Geometry: final body of the model. Coordinates: model frame, mm. A direction names the side the tool comes from. Round coordinates to 2 decimals unless told otherwise and drop trailing zeros. Order: outer loops, then holes, each group sorted by start corner. A loop starts at its lowest first (then second) coordinate and runs counter-clockwise, first axis right, second up. Notation, with made-up numbers: M 88.5,51 L 103.5,51 A12 ccw 103.5,61 Z; hole C 0.5,14.5 d8. An arc over 180 degrees is marked long. Put each result on its own line as item: value. Start each with the question number.
1) Section A-A, the plane y = 3.25. Return loops of the section in (x, z), then the cut area to 3 significant figures.
2) Access query for faces 1 (the flat face through (-10, 3, -16.75)), 2 (the flat face through (-2, 3, -10)), 3 (the flat face through (-10, 3, -2)). Directions: +Z, -Z, +X, -X, +Y, -Y. A direction counts if a zero-diameter tool reaches every point of the face in a straight line with its end or side. Return the directions, or none.
3) Material intervals for probe 1 along X at (y, z) = (2.5, -13.5); probe 2 along Z at (x, y) = (-10, 6.5), sorted ascending. Write a range as [from, to].
4) First-contact query: P1, Ø3, axis at y = 7.5, z = -12.5, coming from the -X side; P2, Ø2, axis at x = -7.5, y = 6, coming from the -Z side; P3, Ø1.5, axis at x = -8, y = 7, coming from the +Z side. Flat tips, straight axial feed; report the tip coordinate or a pass-through.
5) Section D-D, the plane y = 6.5. Return loops of the section in (x, z).
6) Section C-C, the plane z = -13.75. Return loops of the section in (x, y).
7) Draft query along X for faces 4 (the flat face through (-6, 7, -10)), 5 (the flat face through (-18, 3, -10)), 6 (the flat face through (-10, 2, -19)). Return one class per face: pulls with the +X half, pulls with the -X half, needs draft (parallel to the pull), parting line crosses it, or undercut.
8) Section B-B, the plane x = -5.75. Return loops of the section in (y, z), then the cut area to 3 significant figures.
Autodesk Inventor part; units mm, degrees
ref_plane "YZ Plane" through (0, 0, 0) normal (1, 0, 0) x (0, 1, 0)
ref_plane "XZ Plane" through (0, 0, 0) normal (0, 1, 0) x (-1, 0, 0)
ref_plane "XY Plane" through (0, 0, 0) normal (0, 0, 1) x (1, 0, 0)
sketch "Sketch1" plane through (0, 0, 0) normal (0, 1, 0) x (-1, 0, 0)
  line L0 (0, 0) -> (20, 0)
  line L1 (20, 0) -> (20, -20)
  line L2 (20, -20) -> (0, -20)
  line L3 (0, -20) -> (0, 0)
  dimension "d0" = 20
  dimension "d1" = 20
extrude "Extrusion1" add sketch "Sketch1" along normal blind 2
sketch "Sketch2" plane through (0, 2, 0) normal (0, 1, 0) x (1, 0, 0)
  line L0 (0, 20) -> (-20, 20)
  line L1 (-20, 20) -> (-20, 0)
  line L2 (-20, 0) -> (0, 0)
  line L3 (0, 0) -> (0, 20)
  line L4 (-18, 2) -> (-18, 18)
  line L5 (-18, 18) -> (-2, 18)
  line L6 (-2, 18) -> (-2, 2)
  line L7 (-2, 2) -> (-18, 2)
  line L8 (-16.75, 16.75) -> (-16.75, 3.25)
  line L9 (-16.75, 3.25) -> (-3.25, 3.25)
  line L10 (-3.25, 3.25) -> (-3.25, 16.75)
  line L11 (-3.25, 16.75) -> (-16.75, 16.75)
  dimension "d4" = 2
  dimension "d5" = 1.25
extrude "Extrusion2" add sketch "Sketch2" along normal blind 2 contours L4 L5 L6 L7
extrude "Extrusion3" cut sketch "Sketch2" against normal blind 10 contours L11 L10 L9 L8
sketch "Sketch3" plane through (0, 0, 0) normal (0, -1, 0) x (1, 0, 0)
  line L0 (-3.25, -3.25) -> (-3.25, -16.75)
  line L1 (-3.25, -16.75) -> (-16.75, -16.75)
  line L2 (-16.75, -16.75) -> (-16.75, -3.25)
  line L3 (-16.75, -3.25) -> (-3.25, -3.25)
  line L4 (0, -20) -> (-20, -20)
  line L5 (0, 0) -> (0, -20)
  line L6 (-20, 0) -> (0, 0)
  line L7 (-20, -20) -> (-20, 0)
  line L8 (-6, -6) -> (-6, -14)
  line L9 (-6, -14) -> (-14, -14)
  line L10 (-14, -14) -> (-14, -6)
  line L11 (-14, -6) -> (-6, -6)
extrude "Extrusion4" add sketch "Sketch3" against normal up to surface (2 mm away) contours L0 L1 L2 L3
extrude "Extrusion5" add sketch "Sketch3" against normal blind 12.5 contours L8 L9 L10 L11
properties part number "latticeChamberCapv4"
Result sheet:
1. outline: M -18,-18 L -2,-18 L -2,-2 L -18,-2 Z; M -14,-14 L -6,-14 L -6,-6 L -14,-6 Z; hole M -16.75,-16.75 L -3.25,-16.75 L -3.25,-3.25 L -16.75,-3.25 Z
1. area: 138 mm2
2. face 1: +Y
2. face 2: +Z, -Z, +X, +Y
2. face 3: +Z, +X, -X, +Y
3. probe 1: x = [-18, -16.75], [-14, -6], [-3.25, -2]
3. probe 2: z = [-14, -6]
4. P1: stops at x = -14
4. P2: stops at z = -14
4. P3: stops at z = -6
5. outline: M -14,-14 L -6,-14 L -6,-6 L -14,-6 Z
6. outline: M -20,0 L 0,0 L 0,2 L -2,2 L -2,4 L -3.25,4 L -3.25,2 L -6,2 L -6,12.5 L -14,12.5 L -14,2 L -16.75,2 L -16.75,4 L -18,4 L -18,2 L -20,2 Z
7. face 4: undercut
7. face 5: pulls with the -X half
7. face 6: needs draft
8. outline: M 0,-20 L 2,-20 L 2,-18 L 4,-18 L 4,-16.75 L 2,-16.75 L 2,-3.25 L 4,-3.25 L 4,-2 L 2,-2 L 2,0 L 0,0 Z
8. area: 45.0 mm2
